```python
from build123d import *

# Parameters (mm, degrees)
SKETCH_1_R               = 13
EXTRUDE_1_DEPTH          = 4
SKETCH_2_W               = 84
SKETCH_2_H               = 62
EXTRUDE_2_DEPTH          = 4
SKETCH_3_R               = 4.5
CUT_EXTRUDE_1_DEPTH      = 10
SKETCH_4_R               = 1.5
CUT_EXTRUDE_2_DEPTH      = 123.494897853
SKETCH_8_W               = 18
SKETCH_8_H               = 44
EXTRUDE_4_DEPTH          = 4
SKETCH_9_W               = 64
SKETCH_9_H               = 22
CUT_EXTRUDE_6_DEPTH      = 130.772878522
SKETCH_10_R              = 1.5
CUT_EXTRUDE_7_DEPTH      = 130.772878522
SKETCH_11_R              = 1.5
CUT_EXTRUDE_8_DEPTH      = 130.772878522
SKETCH_12_R              = 1.5
CUT_EXTRUDE_9_DEPTH      = 130.772878522
FILLET_1_R               = 3
SKETCH_13_W              = 20
SKETCH_13_H              = 18
CUT_EXTRUDE_10_DEPTH     = 130.772878522
FILLET_2_R               = 3
PATTERN_CIRCULAR_1_COUNT = 3
SKETCH_15_W              = 125.49724571
SKETCH_15_H              = 54.116042209
CUT_EXTRUDE_11_DEPTH     = 130.772878522
FILLET_3_R               = 3
SKETCH_16_R              = 1.5
CUT_EXTRUDE_12_DEPTH     = 97.13012015
SKETCH_17_W              = 168.959633348
SKETCH_17_H              = 62.358711946
CUT_EXTRUDE_13_DEPTH     = 97.13012015
FILLET_4_R               = 1


with BuildPart() as part:
    # 草图1 → 凸台-拉伸1 (new body)
    with BuildSketch(Plane.XY):
        with BuildLine():
            ThreePointArc((34.722027765, 4.402361625), (0, 35), (-34.722027765, 4.402361625))
            Line((-34.722027765, 4.402361625), (-42, -53))
            Line((-42, -53), (42, -53))
            Line((42, -53), (34.722027765, 4.402361625))
        make_face()
        Circle(SKETCH_1_R, mode=Mode.SUBTRACT)
    extrude(amount=EXTRUDE_1_DEPTH)

    # 草图2 → 凸台-拉伸2 (add)
    with BuildSketch(Plane.XY.offset(4)):
        with Locations((0, -84)):
            Rectangle(SKETCH_2_W, SKETCH_2_H)
    extrude(amount=-EXTRUDE_2_DEPTH)

    # 草图3 → 切除-拉伸1 (cut)
    with BuildSketch(Plane.XY.offset(4)):
        with Locations((0, 22.5)):
            Circle(SKETCH_3_R)
    cut_extrude_1 = extrude(amount=-CUT_EXTRUDE_1_DEPTH, mode=Mode.SUBTRACT)

    # 草图4 → 切除-拉伸2 (cut, through all)
    with BuildSketch(Plane.XY.offset(4)):
        with Locations((15.155444566, 8.75)):
            Circle(SKETCH_4_R)
        with Locations((0, -17.5)):
            Circle(SKETCH_4_R)
        with Locations((-15.155444566, 8.75)):
            Circle(SKETCH_4_R)
    extrude(amount=-CUT_EXTRUDE_2_DEPTH, mode=Mode.SUBTRACT)

    # 草图8 → 凸台-拉伸4 (add)
    with BuildSketch(Plane.XY.offset(4)):
        with Locations((-51, -75)):
            Rectangle(SKETCH_8_W, SKETCH_8_H)
    extrude_4 = extrude(amount=-EXTRUDE_4_DEPTH)

    # 镜向3: 凸台-拉伸4 across plane
    add(extrude_4.mirror(Plane(origin=(0, 0, 0), x_dir=(0, 0, 1), z_dir=(1, 0, 0))))

    # 草图9 → 切除-拉伸6 (cut, through all)
    with BuildSketch(Plane(origin=(0, 0, 0), x_dir=(-1, 0, 0), z_dir=(0, 0, -1))):
        with Locations((0, -76)):
            Rectangle(SKETCH_9_W, SKETCH_9_H)
    extrude(amount=-CUT_EXTRUDE_6_DEPTH, mode=Mode.SUBTRACT)

    # 草图10 → 切除-拉伸7 (cut, through all)
    with BuildSketch(Plane(origin=(0, 0, 0), x_dir=(-1, 0, 0), z_dir=(0, 0, -1))):
        with Locations((0, -107.5)):
            Circle(SKETCH_10_R)
        with Locations((24, -107.5)):
            Circle(SKETCH_10_R)
    cut_extrude_7 = extrude(amount=-CUT_EXTRUDE_7_DEPTH, mode=Mode.SUBTRACT)

    # 镜向4: 切除-拉伸7 across plane
    add(cut_extrude_7.mirror(Plane(origin=(0, 0, 0), x_dir=(0, 0, 1), z_dir=(1, 0, 0))), mode=Mode.SUBTRACT)

    # 草图11 → 切除-拉伸8 (cut, through all)
    with BuildSketch(Plane(origin=(0, 0, 0), x_dir=(-1, 0, 0), z_dir=(0, 0, -1))):
        with Locations((-52.5, -67.5)):
            Circle(SKETCH_11_R)
        with Locations((-52.5, -90)):
            Circle(SKETCH_11_R)
    cut_extrude_8 = extrude(amount=-CUT_EXTRUDE_8_DEPTH, mode=Mode.SUBTRACT)

    # 镜向5: 切除-拉伸8 across plane
    add(cut_extrude_8.mirror(Plane(origin=(0, 0, 0), x_dir=(0, 0, 1), z_dir=(1, 0, 0))), mode=Mode.SUBTRACT)

    # 草图12 → 切除-拉伸9 (cut, through all)
    with BuildSketch(Plane(origin=(0, 0, 0), x_dir=(-1, 0, 0), z_dir=(0, 0, -1))):
        with Locations((-30, -36)):
            Circle(SKETCH_12_R)
    cut_extrude_9 = extrude(amount=-CUT_EXTRUDE_9_DEPTH, mode=Mode.SUBTRACT)

    # 镜向6: 切除-拉伸9 across plane
    add(cut_extrude_9.mirror(Plane(origin=(0, 0, 0), x_dir=(0, 0, 1), z_dir=(1, 0, 0))), mode=Mode.SUBTRACT)

    # 圆角1
    fillet_1_edges = [part.edges().sort_by_distance(p)[0] for p in [
        (42, -53, 2),
        (-42, -53, 2),
        (-42, -97, 2),
        (42, -97, 2),
        (-32, -65, 2),
        (-32, -87, 2),
        (32, -87, 2),
        (32, -65, 2),
    ]]
    fillet(fillet_1_edges, radius=FILLET_1_R)

    # 草图13 → 切除-拉伸10 (cut, through all)
    with BuildSketch(Plane(origin=(0, 0, 0), x_dir=(-1, 0, 0), z_dir=(0, 0, -1))):
        with Locations((50, -106)):
            Rectangle(SKETCH_13_W, SKETCH_13_H)
    cut_extrude_10 = extrude(amount=-CUT_EXTRUDE_10_DEPTH, mode=Mode.SUBTRACT)

    # 镜向7: 切除-拉伸10 across plane
    add(cut_extrude_10.mirror(Plane(origin=(0, 0, 0), x_dir=(0, 0, 1), z_dir=(1, 0, 0))), mode=Mode.SUBTRACT)

    # 圆角2
    fillet_2_edges = [part.edges().sort_by_distance(p)[0] for p in [
        (-40, -97, 2),
        (40, -97, 2),
    ]]
    fillet(fillet_2_edges, radius=FILLET_2_R)

    # 阵列(圆周)1: 切除-拉伸1 ×3 about axis
    pattern_circular_1_axis = Axis((0, 0, 0), (0, 0, 1))
    for i in range(1, PATTERN_CIRCULAR_1_COUNT):
        add(cut_extrude_1.rotate(pattern_circular_1_axis, i * 360 / PATTERN_CIRCULAR_1_COUNT), mode=Mode.SUBTRACT)

    # 草图15 → 切除-拉伸11 (cut, through all)
    with BuildSketch(Plane.XY.offset(4)):
        with Locations((2.748622855, -102.058021104)):
            Rectangle(SKETCH_15_W, SKETCH_15_H)
    extrude(amount=-CUT_EXTRUDE_11_DEPTH, mode=Mode.SUBTRACT)

    # 圆角3
    fillet_3_edges = [part.edges().sort_by_distance(p)[0] for p in [
        (32, -75, 2),
        (-32, -75, 2),
    ]]
    fillet(fillet_3_edges, radius=FILLET_3_R)

    # 草图16 → 切除-拉伸12 (cut, through all)
    with BuildSketch(Plane(origin=(0, 0, 0), x_dir=(-1, 0, 0), z_dir=(0, 0, -1))):
        with Locations((0, -36)):
            Circle(SKETCH_16_R)
    extrude(amount=-CUT_EXTRUDE_12_DEPTH, mode=Mode.SUBTRACT)

    # 草图17 → 切除-拉伸13 (cut, through all)
    with BuildSketch(Plane(origin=(0, 0, 0), x_dir=(-1, 0, 0), z_dir=(0, 0, -1))):
        with Locations((4.236961123, -74.679355973)):
            Rectangle(SKETCH_17_W, SKETCH_17_H)
    extrude(amount=-CUT_EXTRUDE_13_DEPTH, mode=Mode.SUBTRACT)

    # 圆角4
    fillet_4_edges = [part.edges().sort_by_distance(p)[0] for p in [
        (40.795507114, -43.5, 2),
        (-40.795507114, -43.5, 2),
    ]]
    fillet(fillet_4_edges, radius=FILLET_4_R)


solid = part.part
```
Work out the finished part from the listing and answer in its coordinate system (mm). Coordinates: 2 decimals unless noted, no trailing zeros. Loops run counter-clockwise (first coordinate to the right, second up) from the corner with the lowest first, then second, coordinate; pieces in that order, holes last. Notation, with made-up numbers: (56, 29) - (61, 29) arc R8 ccw to (61, 35) - close; hole circle Ø10 at (11, 13.5). An arc over 180 degrees is marked (long way). Use a Markdown table: item, result.
Item 1: Consider probe 1 along Y at (x, z) = (16, 1); probe 2 along Y at (x, z) = (0, 0.9); probe 3 along X at (y, z) = (-2, 2.3). Determine where each line is inside the solid, lowest interval first. Write a range as from..to.
Evaluation:
| item | result |
|---|---|
| probe 1 | y = -43.5..-14.1, -8.4..7.51, 9.99..31.13 |
| probe 2 | y = -43.5..-37.5, -34.5..-19, -16..-13, 13..18, 27..35 |
| probe 3 | x = -35.53..-12.85, 12.85..35.53 |
Item 2: The mould has two halves that part along X. Classify faces 1 (the flat face through (37.73, -19.31, 1.97)), 2 (the cylindrical face through (-0.59, 26.96, 2.03)), 3 (the cylindrical face through (31.2, -36.9, 2)), 4 (the flat face through (-8, -12, 4)): +X half, -X half, draft (parallel to the pull), parting line (faces both ways), or undercut.
Evaluation:
| item | result |
|---|---|
| face 1 | +X half |
| face 2 | undercut |
| face 3 | undercut |
| face 4 | draft |
Item 3: Given pin 1 Ø2 at (y, z) = (0, 0.5) entering from +X, flat-ended and moving along its own axis, determine where the tip first touches the part or whether it passes through.
Evaluation:
| item | result |
|---|---|
| pin 1 | stops at x = 35.41 |
Item 4: Find section D-D, the plane z = 2.55. State how many separate pieces and enclosed holes the cut face has, and give its area (3 significant figures).
Evaluation:
| item | result |
|---|---|
| separate pieces | 1 |
| enclosed holes | 10 |
| area | 4,470 mm2 |
Item 5: Find section B-B, the plane y = -17.5. Determine the outline of the cut face in (x, z).
Evaluation:
| item | result |
|---|---|
| outline | (-37.5, 0) - (-1.5, 0) - (-1.5, 4) - (-37.5, 4) - close; (1.5, 0) - (37.5, 0) - (37.5, 4) - (1.5, 4) - close |
Item 6: Find section C-C, the plane x = -20. Determine the outline of the cut face in (y, z), and give its area (3 significant figures).
Evaluation:
| item | result |
|---|---|
| outline | (-43.5, 0) - (-15.72, 0) - (-15.72, 4) - (-43.5, 4) - close; (-6.78, 0) - (28.72, 0) - (28.72, 4) - (-6.78, 4) - close |
| area | 253 mm2 |
Item 7: Find section A-A, the plane x = 0. Determine the outline of the cut face in (y, z).
Evaluation:
| item | result |
|---|---|
| outline | (-43.5, 0) - (-37.5, 0) - (-37.5, 4) - (-43.5, 4) - close; (-34.5, 0) - (-19, 0) - (-19, 4) - (-34.5, 4) - close; (-16, 0) - (-13, 0) - (-13, 4) - (-16, 4) - close; (13, 0) - (18, 0) - (18, 4) - (13, 4) - close; (27, 0) - (35, 0) - (35, 4) - (27, 4) - close |
